from build123d import *

# Parameters (mm, degrees)
SKETCH1_W           = 203.2
SKETCH1_H           = 50.8
SKETCH1_R           = 3.175
BOSS_EXTRUDE1_DEPTH = 6.35


with BuildPart() as part:
    # Sketch1 → Boss-Extrude1 (new body)
    with BuildSketch(Plane(origin=(0, 0, 0), x_dir=(1, 0, 0), z_dir=(0, 1, 0))):
        Rectangle(SKETCH1_W, SKETCH1_H)
        with Locations(Location((-88.9, 12.7, 0), (0, 0, 270))):
            Circle(SKETCH1_R, mode=Mode.SUBTRACT)
        with Locations(Location((-63.5, 12.7, 0), (0, 0, 270))):
            Circle(SKETCH1_R, mode=Mode.SUBTRACT)
        with Locations(Location((-38.1, 12.7, 0), (0, 0, 270))):
            Circle(SKETCH1_R, mode=Mode.SUBTRACT)
        with Locations(Location((-12.7, 12.7, 0), (0, 0, 270))):
            Circle(SKETCH1_R, mode=Mode.SUBTRACT)
        with Locations(Location((12.7, 12.7, 0), (0, 0, 270))):
            Circle(SKETCH1_R, mode=Mode.SUBTRACT)
        with Locations(Location((38.1, 12.7, 0), (0, 0, 270))):
            Circle(SKETCH1_R, mode=Mode.SUBTRACT)
        with Locations(Location((63.5, 12.7, 0), (0, 0, 270))):
            Circle(SKETCH1_R, mode=Mode.SUBTRACT)
        with Locations(Location((88.9, 12.7, 0), (0, 0, 270))):
            Circle(SKETCH1_R, mode=Mode.SUBTRACT)
        with Locations(Location((-63.5, -12.7, 0), (0, 0, 270))):
            Circle(SKETCH1_R, mode=Mode.SUBTRACT)
        with Locations(Location((-38.1, -12.7, 0), (0, 0, 270))):
            Circle(SKETCH1_R, mode=Mode.SUBTRACT)
        with Locations(Location((-12.7, -12.7, 0), (0, 0, 270))):
            Circle(SKETCH1_R, mode=Mode.SUBTRACT)
        with Locations(Location((12.7, -12.7, 0), (0, 0, 270))):
            Circle(SKETCH1_R, mode=Mode.SUBTRACT)
        with Locations(Location((38.1, -12.7, 0), (0, 0, 270))):
            Circle(SKETCH1_R, mode=Mode.SUBTRACT)
        with Locations(Location((63.5, -12.7, 0), (0, 0, 270))):
            Circle(SKETCH1_R, mode=Mode.SUBTRACT)
        with Locations(Location((88.9, -12.7, 0), (0, 0, 270))):
            Circle(SKETCH1_R, mode=Mode.SUBTRACT)
        with Locations(Location((-88.9, -12.7, 0), (0, 0, 270))):
            Circle(SKETCH1_R, mode=Mode.SUBTRACT)
    extrude(amount=BOSS_EXTRUDE1_DEPTH)


solid = part.part
Can you work these out from the model? Positions are in its coordinate system, mm. Give positions to 0.01 mm unless a question says otherwise; leave off trailing zeros. Loops run counter-clockwise (first coordinate to the right, second up) from the corner with the lowest first, then second, coordinate; pieces in that order, holes last. Notation, with made-up numbers: (-17.75, 82.5) -> (4.25, 82.5) arc R21 ccw to (4.25, 111.5) -> close; hole circle Ø5 at (66, 75.5). An arc over 180 degrees is marked (long way). Use one line per item in the form item = value.
1) We'd pull the mould along X, two halves only. Please class faces 1 (the face through (-101.6, 3, 0)), 2 (the face through (-1, 3, -25.4)), 3 (the face through (9.9, 3.1, -11.2)): released by +X, released by -X, zero draft, split by the parting line, or undercut.
Answers:
face_1 = released by -X
face_2 = zero draft
face_3 = undercut
2) If we section it at B-B (y = 1.75): Count the separate pieces of the cut face and the enclosed holes in it, plus the area to 3 significant figures.
Answers:
separate_pieces = 1
enclosed_holes = 16
area = 9,820 mm²
3) If we section it at A-A (x = -12.7): Please give me the cut outline in (y, z) (3 decimals), plus the area to 3 significant figures.
Answers:
outline = (0, -25.4) -> (6.35, -25.4) -> (6.35, -15.875) -> (0, -15.875) -> close; (0, -9.525) -> (6.35, -9.525) -> (6.35, 9.525) -> (0, 9.525) -> close; (0, 15.875) -> (6.35, 15.875) -> (6.35, 25.4) -> (0, 25.4) -> close
area = 242 mm²
4) I need wall thicknesses on line 1 along Z through (x, y) = (61.5, 4.5); line 2 along Z through (x, y) = (-90.5, 2.5). Which ranges of each line are inside material? Lowest first, please.
Answers:
line_1 = -25.4 to -15.17, -10.23 to 10.23, 15.17 to 25.4
line_2 = -25.4 to -15.44, -9.96 to 9.96, 15.44 to 25.4
